Study the drawing (mm; zero at the part's minimum x, y, z) and answer. Round coordinates to 2 decimals unless told otherwise and drop trailing zeros. Order: outer loops, then holes, each group sorted by start corner. A loop starts at its lowest first (then second) coordinate and runs counter-clockwise, first axis right, second up. Notation, with made-up numbers: M -20.5,45 L -9.5,45 A24 ccw -9.5,72 Z; hole C 19,-10 d9. An arc over 180 degrees is marked long. Put each result on its own line as item: value. Start each with the question number.
1. The part is cut by section B-B (y = 39). Give the vertices of the cut face in (x, z), then the cut area to 3 significant figures.
2. Each of these flat-tipped pins is pushed along its axis until it touches: pin 1 Ø0.6 at (y, z) = (2, 1) entering from -X; pin 2 Ø0.6 at (y, z) = (44, 0.5) entering from +X; pin 3 Ø1 at (x, z) = (1, 1) entering from +Y. Where does it stop, or does it pass through?
3. The part is cut by section C-C (x = 17.5). Give the vertices of the cut face in (y, z), then the cut area to 3 significant figures.
4. The part is cut by section A-A (z = 1.2). Give the vertices of the cut face in (x, y), then the cut area to 3 significant figures.
5. Consider line 1 (X direction, y = 43.5, z = 0.7); line 2 (X direction, y = 7, z = 1.4); line 3 (Y direction, x = 30, z = 1) (3 decimals). Determine where each line is inside the solid, lowest interval first.
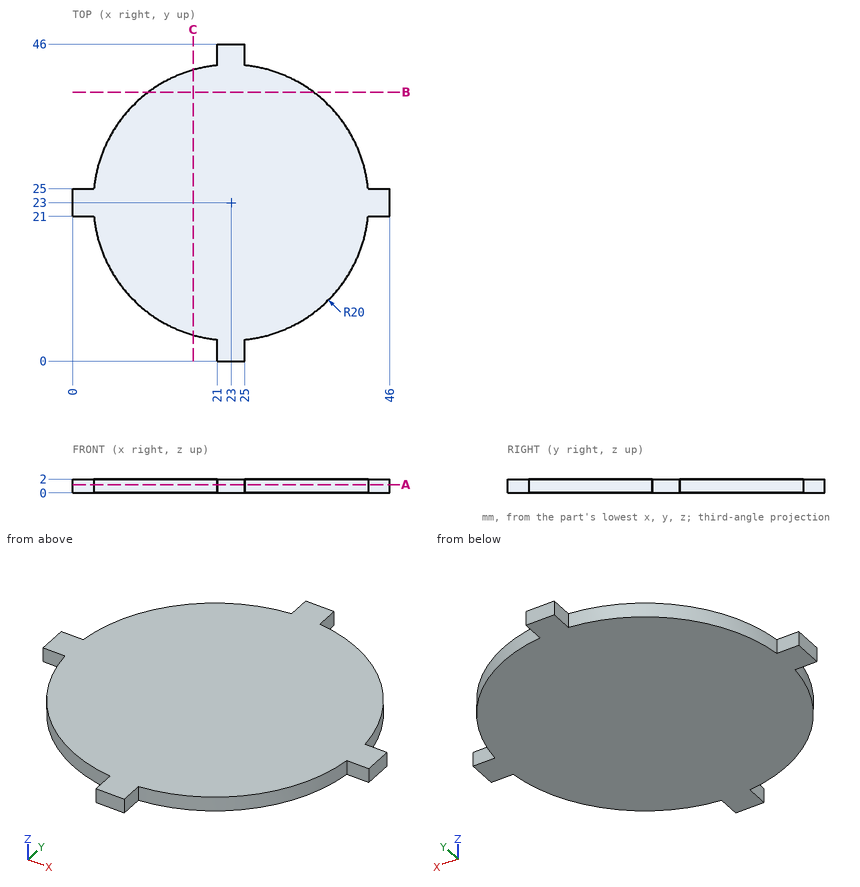
Resolved:
1. outline: M 11,0 L 35,0 L 35,2 L 11,2 Z
1. area: 48.0 mm2
2. pin 1: x = 21
2. pin 2: x = 25
2. pin 3: y = 25
3. outline: M 3.77,0 L 42.23,0 L 42.23,2 L 3.77,2 Z
3. area: 76.9 mm2
4. outline: M 0,21 L 3.1,21 A20 ccw 21,3.1 L 21,0 L 25,0 L 25,3.1 A20 ccw 42.9,21 L 46,21 L 46,25 L 42.9,25 A20 ccw 25,42.9 L 25,46 L 21,46 L 21,42.9 A20 ccw 3.1,25 L 0,25 Z
4. area: 1,310 mm2
5. line 1: 21 to 25
5. line 2: 11 to 35
5. line 3: 4.265 to 41.735
